from build123d import *

# Parameters (mm, degrees)
SKETCH1_W           = 25
SKETCH1_H           = 38
BOSS_EXTRUDE1_DEPTH = 122
SKETCH2_W           = 80
SKETCH2_H           = 24
CUT_EXTRUDE1_DEPTH  = 22.5
FILLET1_R           = 6
FILLET2_R           = 6
FILLET3_R           = 6
FILLET4_R           = 6
SKETCH3_R           = 9.2
CUT_EXTRUDE2_DEPTH  = 126.503984001
CHAMFER2_SIZE       = 2


with BuildPart() as part:
    # Sketch1 → Boss-Extrude1 (new body)
    with BuildSketch(Plane(origin=(0, 0, 0), x_dir=(0, 0, -1), z_dir=(1, 0, 0))):
        Rectangle(SKETCH1_W, SKETCH1_H)
    extrude(amount=BOSS_EXTRUDE1_DEPTH)

    # Sketch2 → Cut-Extrude1 (cut)
    with BuildSketch(Plane.XY.offset(12.5)):
        with Locations((43, 0)):
            Rectangle(SKETCH2_W, SKETCH2_H)
    extrude(amount=-CUT_EXTRUDE1_DEPTH, mode=Mode.SUBTRACT)

    # Fillet1
    fillet1_edges = [part.edges().sort_by_distance(p)[0] for p in [
        (3, 12, 1.25),
    ]]
    fillet(fillet1_edges, radius=FILLET1_R)

    # Fillet2
    fillet2_edges = [part.edges().sort_by_distance(p)[0] for p in [
        (3, -12, 1.25),
    ]]
    fillet(fillet2_edges, radius=FILLET2_R)

    # Fillet3
    fillet3_edges = [part.edges().sort_by_distance(p)[0] for p in [
        (83, -12, 1.25),
    ]]
    fillet(fillet3_edges, radius=FILLET3_R)

    # Fillet4
    fillet4_edges = [part.edges().sort_by_distance(p)[0] for p in [
        (83, 12, 1.25),
    ]]
    fillet(fillet4_edges, radius=FILLET4_R)

    # Sketch3 → Cut-Extrude2 (cut, through all)
    with BuildSketch(Plane.XY.offset(-10)):
        with Locations((43, 0)):
            Circle(SKETCH3_R)
    extrude(amount=-CUT_EXTRUDE2_DEPTH, mode=Mode.SUBTRACT)

    # Chamfer2
    chamfer2_edges = [part.edges().sort_by_distance(p)[0] for p in [
        (122, 0, -12.5),
        (0, 0, -12.5),
        (61, -19, -12.5),
        (61, 19, -12.5),
    ]]
    chamfer(chamfer2_edges, length=CHAMFER2_SIZE)


solid = part.part
For this review, take the finished solid that the model builds, in its own axes (mm). A direction names the side the tool comes from. Give positions to 0.01 mm unless a question says otherwise; leave off trailing zeros. Order: outer loops, then holes, each group sorted by start corner. A loop starts at its lowest first (then second) coordinate and runs counter-clockwise, first axis right, second up. Notation, with made-up numbers: (-32, 67.25) - (7, 67.25) arc R27 ccw to (7, 101.25) - close; hole circle Ø3 at (-7, 52.5). An arc over 180 degrees is marked (long way). Answer as a JSON object with one key per item and string values. Group by question number.
Item 1: Machinability: for faces 4 (the cylindrical face through (4.804, 10.289, 1.092)), 5 (the flat face through (74, -13, 12.5)), which of the approach directions +Z, -Z, +X, -X, +Y, -Y give a long, thin tool a straight path to every point of the face, cutting with its end or side? Answer none if there is none.
Item 2: Take a section at D-D on x = 63.5. Give the boundary of the cut face in (y, z).
Item 3: Take a section at B-B on y = 0. Give the boundary of the cut face in (x, z).
Item 4: Clearance check with flat-ended pins moving along their axes: pin 1 Ø5 at (x, y) = (81.5, -2) entering from +Z; pin 2 Ø7 at (x, y) = (58.5, -1.5) entering from +Z; pin 3 Ø14.5 at (x, y) = (43, 0) entering from +Z. State where each tip first meets the part, or that it passes through.
Item 5: Draft analysis for pull direction Y (two halves, no side actions). For faces 1 (the flat face through (0, 0, 1)), 2 (the cylindrical face through (81.289, 10.196, 1.092)), 3 (the flat face through (60.1, 18, -11.5)), state which applies: pulls with the +Y half, pulls with the -Y half, needs draft (parallel to the pull), parting line crosses it, or undercut.
Item 6: Take a section at C-C on x = 43. Give the boundary of the cut face in (y, z), and give its area (3 significant figures).
Item 7: Take a section at A-A on z = 7. Give the boundary of the cut face in (x, y).
Item 8: Wall thickness on line 1 along Y through (x, z) = (45, 3.5); line 2 along X through (y, z) = (-6, 7.75); line 3 along Z through (x, y) = (49, 17.5): over which ranges is each line inside the solid? List them lowest first.
Reported:
{
 "1": {"face 4": "+Z", "face 5": "+Z, +X, -X, +Y, -Y"},
 "2": {"outline": "(-19, -10.5) - (-17, -12.5) - (17, -12.5) - (19, -10.5) - (19, 12.5) - (12, 12.5) - (12, -10) - (-12, -10) - (-12, 12.5) - (-19, 12.5) - close"},
 "3": {"outline": "(0, -10.5) - (2, -12.5) - (33.8, -12.5) - (33.8, -10) - (3, -10) - (3, 12.5) - (0, 12.5) - close; (52.2, -12.5) - (120, -12.5) - (122, -10.5) - (122, 12.5) - (83, 12.5) - (83, -10) - (52.2, -10) - close"},
 "4": {"pin 1": "z = 12.5", "pin 2": "z = -10", "pin 3": "through"},
 "5": {"face 1": "needs draft", "face 2": "undercut", "face 3": "pulls with the +Y half"},
 "6": {"outline": "(-19, -10.5) - (-17, -12.5) - (-9.2, -12.5) - (-9.2, -10) - (-12, -10) - (-12, 12.5) - (-19, 12.5) - close; (9.2, -12.5) - (17, -12.5) - (19, -10.5) - (19, 12.5) - (12, 12.5) - (12, -10) - (9.2, -10) - close", "area": "360 mm^2"},
 "7": {"outline": "(0, -19) - (122, -19) - (122, 19) - (0, 19) - close; hole (3, -6) arc R6 ccw to (9, -12) - (77, -12) arc R6 ccw to (83, -6) - (83, 6) arc R6 ccw to (77, 12) - (9, 12) arc R6 ccw to (3, 6) - close"},
 "8": {"line 1": "-19 to -12, 12 to 19", "line 2": "0 to 3, 83 to 122", "line 3": "-12 to 12.5"}
}
